```python
from build123d import *

# Parameters (mm, degrees)
F3_DEPTH      = 3.81
F3_DEPTH_BACK = 3.81
F4_T4_DEPTH   = 81.9290237066
F4_T9_DEPTH   = 81.9290237066
F4_T14_DEPTH  = 81.28
F4_T19_DEPTH  = 81.28


# Not quite as in the source:
# - a fillet or chamfer that OpenCascade refuses, or shapes differently, is made with other operations: its cross-section is extruded or revolved along the edge and cut away or added


with BuildPart() as f1:
    # F0 (on Front) → F1 (revolve)
    with BuildSketch(Plane.XZ):
        with BuildLine():
            Line((0, -6.35), (0, 6.35))
            ThreePointArc((0, 6.35), (-6.35, 0), (0, -6.35))
        make_face()
    revolve(axis=Axis((0, 0, 0), (0, 0, -1)))

    # F2 (on Front) → F3 (join, two sides)
    with BuildSketch(Plane.XZ) as f3_sk:
        Polygon((4.1104733182, -5.9445748625), (-4.1104737839, -5.9445748625), (-4.1104737839, -74.5245748625), (4.1104733182, -75.1735985691), align=None)
    extrude(amount=-F3_DEPTH)
    extrude(f3_sk.sketch, amount=F3_DEPTH_BACK)

    # F4: fillet of radius 5.08 on 4 edges, made by hand


with BuildPart() as f4_tool2:
    # F4_s3 → F4_t4 (new body)
    with BuildSketch(Plane.XY.offset(-87.8735985691)):
        with BuildLine():
            ThreePointArc((4.1104733182, 1.27), (2.6225757666, -2.3221024484), (-0.9695266818, -3.81))
            Line((-0.9695266818, -3.81), (-0.9695266818, -3.9116))
            Line((-0.9695266818, -3.9116), (4.2120733182, -3.9116))
            Line((4.2120733182, -3.9116), (4.2120733182, 1.27))
            Line((4.2120733182, 1.27), (4.1104733182, 1.27))
        make_face()
    extrude(amount=F4_T4_DEPTH)

    split(bisect_by=Plane(origin=(-5.8725507458, 0, -74.3854631875), x_dir=(0, 1, 0), z_dir=(0.0787026743, 0, 0.9968981337)), keep=Keep.TOP)


with BuildPart() as f1_1:
    add(f1.part)

    # F4_t1: cut F4_tool2
    add(f4_tool2.part, mode=Mode.SUBTRACT)


with BuildPart() as f4_tool7:
    # F4_s8 → F4_t9 (new body)
    with BuildSketch(Plane.XY.offset(-87.8735985691)):
        with BuildLine():
            ThreePointArc((4.1104733182, -1.27), (2.6225757666, 2.3221024484), (-0.9695266818, 3.81))
            Line((-0.9695266818, 3.81), (-0.9695266818, 3.9116))
            Line((-0.9695266818, 3.9116), (4.2120733182, 3.9116))
            Line((4.2120733182, 3.9116), (4.2120733182, -1.27))
            Line((4.2120733182, -1.27), (4.1104733182, -1.27))
        make_face()
    extrude(amount=F4_T9_DEPTH)

    split(bisect_by=Plane(origin=(-5.8725507458, 0, -74.3854631875), x_dir=(0, 1, 0), z_dir=(0.0787026743, 0, 0.9968981337)), keep=Keep.TOP)


with BuildPart() as f1_2:
    add(f1_1.part)

    # F4_t6: cut F4_tool7
    add(f4_tool7.part, mode=Mode.SUBTRACT)


with BuildPart() as f4_tool12:
    # F4_s13 → F4_t14 (new body)
    with BuildSketch(Plane.XY.offset(-5.9445748625)):
        with BuildLine():
            ThreePointArc((0.9695262161, -3.81), (-2.6225762323, -2.3221024484), (-4.1104737839, 1.27))
            Line((-4.1104737839, 1.27), (-4.2120737839, 1.27))
            Line((-4.2120737839, 1.27), (-4.2120737839, -3.9116))
            Line((-4.2120737839, -3.9116), (0.9695262161, -3.9116))
            Line((0.9695262161, -3.9116), (0.9695262161, -3.81))
        make_face()
    extrude(amount=-F4_T14_DEPTH)

    split(bisect_by=Plane(origin=(-5.8725507458, 0, -74.3854631875), x_dir=(0, 1, 0), z_dir=(0.0787026743, 0, 0.9968981337)), keep=Keep.TOP)


with BuildPart() as f1_3:
    add(f1_2.part)

    # F4_t11: cut F4_tool12
    add(f4_tool12.part, mode=Mode.SUBTRACT)


with BuildPart() as f4_tool17:
    # F4_s18 → F4_t19 (new body)
    with BuildSketch(Plane.XY.offset(-5.9445748625)):
        with BuildLine():
            ThreePointArc((0.9695262161, 3.81), (-2.6225762323, 2.3221024484), (-4.1104737839, -1.27))
            Line((-4.1104737839, -1.27), (-4.2120737839, -1.27))
            Line((-4.2120737839, -1.27), (-4.2120737839, 3.9116))
            Line((-4.2120737839, 3.9116), (0.9695262161, 3.9116))
            Line((0.9695262161, 3.9116), (0.9695262161, 3.81))
        make_face()
    extrude(amount=-F4_T19_DEPTH)

    split(bisect_by=Plane(origin=(-5.8725507458, 0, -74.3854631875), x_dir=(0, 1, 0), z_dir=(0.0787026743, 0, 0.9968981337)), keep=Keep.TOP)


with BuildPart() as f1_4:
    add(f1_3.part)

    # F4_t16: cut F4_tool17
    add(f4_tool17.part, mode=Mode.SUBTRACT)


solid = f1_4.part
```
Here's how the part is built. I have some questions about the finished solid (model axes, mm). A direction names the side the tool comes from. Coordinates: 2 decimals unless noted, no trailing zeros. Loops run counter-clockwise (first coordinate to the right, second up) from the corner with the lowest first, then second, coordinate; pieces in that order, holes last. Notation, with made-up numbers: (72, 5) -> (116, 5) arc R8 ccw to (116, 20) -> close; hole circle Ø9 at (74.5, 83). An arc over 180 degrees is marked (long way). Return JSON: item names as keys, results as strings.
1) If we section it at B-B, the plane y = 1.25: Write out the boundary of the cut face in (x, z), then the cut area to 3 significant figures.
Results below:
{"outline": "(-3.44, -74.58) -> (3.44, -75.12) -> (3.44, -5.94) -> (1.85, -5.94) arc R6.23 ccw (long way) to (-1.85, -5.94) -> (-3.44, -5.94) -> close", "area": "595 mm²"}
2) If we section it at D-D, the plane x = -5.5: Write out the boundary of the cut face in (y, z).
Results below:
{"outline": "circle Ø6.35 at (0, 0)"}
3) I need wall thicknesses on line 1 (Y direction, x = 0, z = -69); line 2 (Z direction, x = -2, y = -4.75); line 3 (Y direction, x = 2.25, z = -48.5). Which ranges of each line are inside material? Lowest first, please. Write a range as from..to.
Results below:
{"line 1": "-3.72..3.72", "line 2": "-3.71..3.71", "line 3": "-2.66..2.66"}
4) If we section it at C-C, the plane z = -42: Write out the boundary of the cut face in (x, y).
Results below:
{"outline": "(-3.95, 0) arc R5.08 ccw to (0, -3.72) arc R5.08 ccw to (3.95, 0) arc R5.08 ccw to (0, 3.72) arc R5.08 ccw to start"}
5) If we section it at A-A, the plane x = 3: Write out the boundary of the cut face in (y, z).
Results below:
{"outline": "circle Ø11.19 at (0, 0); (-1.9, -75.09) -> (1.9, -75.09) -> (1.9, -5.94) -> (-1.9, -5.94) -> close"}
6) Will these pins go through, and if not, where does the flat tip stop? pin 1 (2 mm diameter, centred on y = -5, z = -50.5, fed in from -X); pin 2 (2 mm diameter, centred on x = -1, y = -0.5, fed in from +Z); pin 3 (4 mm diameter, centred on x = 3.5, z = -29, fed in from -Y); pin 4 (2 mm diameter, centred on y = 0.5, z = -24, fed in from +X).
Results below:
{"pin 1": "through", "pin 2": "z = 6.35", "pin 3": "y = -3.17", "pin 4": "x = 3.95"}
7) For faces 1 (the face through (2.541, -2.402, -41.037)), 2 (the face through (2.541, 2.402, -41.037)), 3 (the face through (-2.48, 2.46, -39.91)), which set-ups out of +Z, -Z, +X, -X, +Y, -Y let a thin tool reach every point of the face, with its end or its side?
Results below:
{"face 1": "-Z, +X, -Y", "face 2": "-Z, +X, +Y", "face 3": "-Z, -X, +Y"}
8) Thinking about a two-plate mould opening in Z: for faces 4 (the face through (-0.055, 0.052, -74.845)), 5 (the face through (-2.48, -2.46, -39.91)), 6 (the face through (2, 2, -5.945)), which applies, +Z half, -Z half, draft (parallel to the pull), parting line (faces both ways), or undercut?
Results below:
{"face 4": "-Z half", "face 5": "draft", "face 6": "undercut"}
